The figure shows three views and two pictorial views of one solid part (mm, origin at its lowest corner). Answer the questions. Give positions to 0.01 mm unless a question says otherwise; leave off trailing zeros. Loops run counter-clockwise (first coordinate to the right, second up) from the corner with the lowest first, then second, coordinate; pieces in that order, holes last.
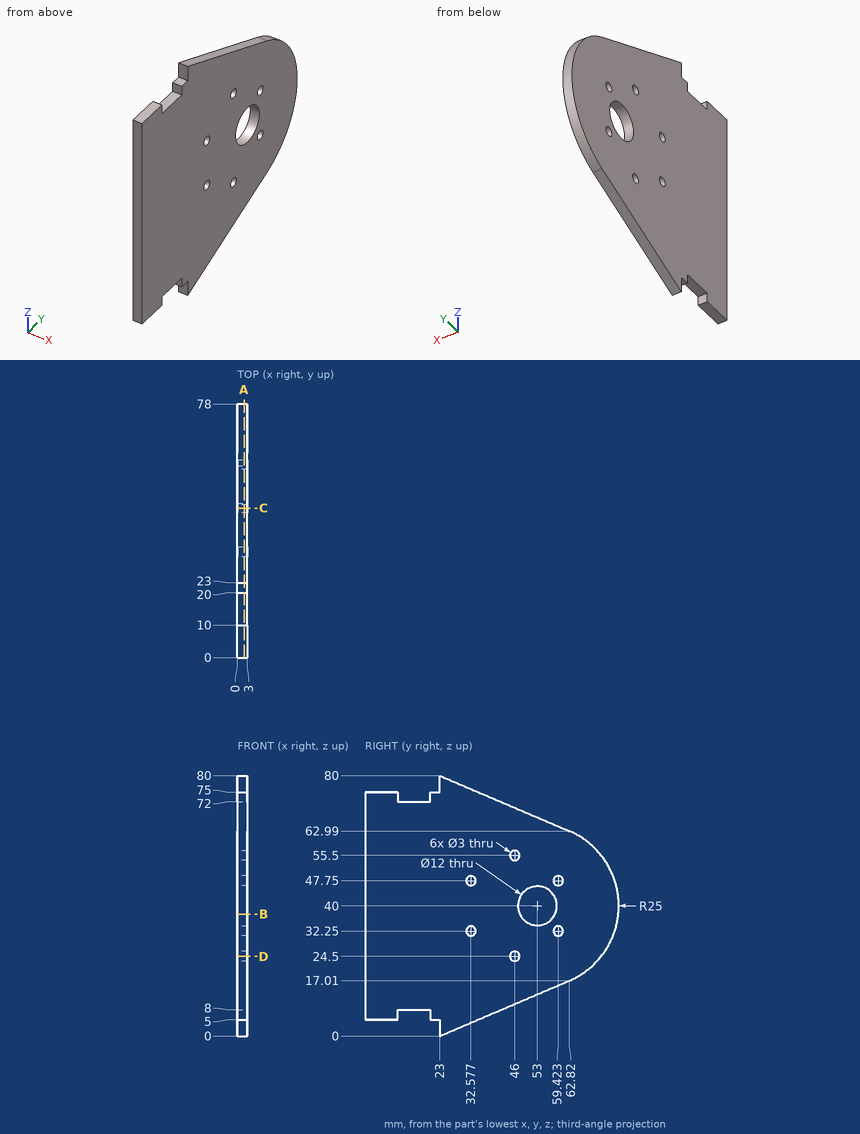
Q1. Given pin 1 (0.9 mm diameter, centred on x = 1, z = 77.5, fed in from -Y); pin 2 (1.5 mm diameter, centred on x = 0.5, z = 28, fed in from +Y) (1 decimal); pin 3 (1.5 mm diameter, centred on x = 1, z = 28.5, fed in from +Y), each flat-ended and moving along its own axis, determine where each tip first touches the part or whether it passes through.
Q2. Section D-D on z = 24.5 is taken. Give the vertices of the cut face in (x, y) (1 decimal), plus the area to 3 significant figures.
Q3. Section A-A on x = 2.1 is taken. Give the vertices of the cut face in (y, z), plus the area to 3 significant figures.
Q4. Section B-B on z = 37.5 is taken. Give the vertices of the cut face in (x, y) (1 decimal), plus the area to 3 significant figures.
Q5. Consider line 1 along Y through (x, z) = (1.9, 39.5) (1 decimal); line 2 along Z through (x, y) = (0.3, 50) (1 decimal); line 3 along Z through (x, y) = (1.2, 21). Determine where each line is inside the solid, lowest interval first.
Q6. Section C-C on y = 46 is taken. Give the vertices of the cut face in (x, z) (1 decimal).
Check result:
1. pin 1: stops at y = 23
1. pin 2: stops at y = 75.3
1. pin 3: stops at y = 75.57
2. outline: (0, 0) - (3, 0) - (3, 44.5) - (0, 44.5) - close; (0, 47.5) - (3, 47.5) - (3, 72.6) - (0, 72.6) - close
2. area: 209 mm2
3. outline: (0, 5) - (10, 5) - (10, 8) - (20, 8) - (20, 5) - (23, 5) - (23, 0) - (62.82, 17.01) arc R25 ccw to (62.82, 62.99) - (23, 80) - (23, 75) - (20, 75) - (20, 72) - (10, 72) - (10, 75) - (0, 75) - close; hole circle Ø3 at (32.58, 32.25); hole circle Ø3 at (32.58, 47.75); hole circle Ø3 at (46, 24.5); hole circle Ø3 at (46, 55.5); hole circle Ø12 at (53, 40); hole circle Ø3 at (59.42, 32.25); hole circle Ø3 at (59.42, 47.75)
3. area: 4,410 mm2
4. outline: (0, 0) - (3, 0) - (3, 47.5) - (0, 47.5) - close; (0, 58.5) - (3, 58.5) - (3, 77.9) - (0, 77.9) - close
4. area: 201 mm2
5. line 1: y = 0 to 47, 59 to 78
5. line 2: z = 11.5 to 34.8, 45.2 to 68.5
5. line 3: z = 5 to 75
6. outline: (0, 9.8) - (3, 9.8) - (3, 23) - (0, 23) - close; (0, 26) - (3, 26) - (3, 54) - (0, 54) - close; (0, 57) - (3, 57) - (3, 70.2) - (0, 70.2) - close
